Here's how the part is built. I have some questions about the finished solid (model axes, mm). Face numbers are marked on the shaded views. A direction names the side the tool comes from. Coordinates: 2 decimals unless noted, no trailing zeros. Write each loop counter-clockwise with the first axis right and the second up, starting at its lowest first coordinate (ties: lowest second). Pieces come first, ordered by that corner, then holes. Notation, with made-up numbers: (40, 23) - (85, 23) arc R21 cw to (85, 54) - close; hole circle Ø6 at (12.25, 11.25). An arc over 180 degrees is marked (long way). Answer in a Markdown table with one row per item. Add a question column.
Item 1: Imagine slicing it at C-C (y = 10.5). Please give me the cut outline in (x, z), plus the area to 3 significant figures.
Item 2: If I drill on probe 1 along X at (y, z) = (4, 4.55); probe 2 along Y at (x, z) = (3.5, 1.65); probe 3 along X at (y, z) = (-3.25, 0.2), over which ranges is the centre line in solid material (lowest first)? Write a range as from..to.
Item 3: Imagine slicing it at A-A (z = 1.5). Please give me the cut outline in (x, y).
Item 4: Which directions (+Z, -Z, +X, -X, +Y, -Y) give clear straight access to the entire face, cutting with the end or side of a thin tool? Please do the marked faces 1, 2 and 3.
Item 5: Imagine slicing it at B-B (x = -7.5). Please give me the cut outline in (y, z).
Item 6: I'm going to push flat-ended pins straight in: pin 1 (0.8 mm diameter, centred on y = 12.5, z = 0.5, fed in from +X); pin 2 (4 mm diameter, centred on x = -3.5, y = 1, fed in from -Z); pin 3 (1.3 mm diameter, centred on y = 10.5, z = 4, fed in from -X); pin 4 (2 mm diameter, centred on y = 9.5, z = 3.5, fed in from +X). Where does each tip first touch, or does it pass through?
from build123d import *

# Parameters (mm, degrees)
BOSS_EXTRUDE1_DEPTH = 5.5
BOSS_EXTRUDE2_DEPTH = 1


with BuildPart() as part:
    # Sketch1 → Boss-Extrude1 (new body)
    with BuildSketch(Plane.XY):
        Polygon((-14.173922558, 7.032133424), (-14.173922558, 1.032133424), (-7.173922558, 1.032133424), (-7.173922558, -5.967866576), (-1.173922558, -5.967866576), (-1.173922558, 1.032133424), (5.826077442, 1.032133424), (5.826077442, 7.032133424), (-1.173922558, 7.032133424), (-1.173922558, 14.032133424), (-7.173922558, 14.032133424), (-7.173922558, 7.032133424), align=None)
    extrude(amount=BOSS_EXTRUDE1_DEPTH)

    # Sketch2 → Boss-Extrude2 (add)
    with BuildSketch(Plane.XY):
        with BuildLine():
            Line((-15.873922558, 8.032133424), (-15.873922558, 0.032133424))
            ThreePointArc((-15.873922558, 0.032133424), (-15.668897304, -0.462841323), (-15.173922558, -0.667866576))
            Line((-15.173922558, -0.667866576), (-10.173922558, -0.667866576))
            ThreePointArc((-10.173922558, -0.667866576), (-9.254683742, -1.048627761), (-8.873922558, -1.967866576))
            Line((-8.873922558, -1.967866576), (-8.873922558, -6.967866576))
            ThreePointArc((-8.873922558, -6.967866576), (-8.668897304, -7.462841323), (-8.173922558, -7.667866576))
            Line((-8.173922558, -7.667866576), (-0.173922558, -7.667866576))
            ThreePointArc((-0.173922558, -7.667866576), (0.321052189, -7.462841323), (0.526077442, -6.967866576))
            Line((0.526077442, -6.967866576), (0.526077442, -1.967866576))
            ThreePointArc((0.526077442, -1.967866576), (0.906838627, -1.048627761), (1.826077442, -0.667866576))
            Line((1.826077442, -0.667866576), (6.826077442, -0.667866576))
            ThreePointArc((6.826077442, -0.667866576), (7.321052189, -0.462841323), (7.526077442, 0.032133424))
            Line((7.526077442, 0.032133424), (7.526077442, 8.032133424))
            ThreePointArc((7.526077442, 8.032133424), (7.321052189, 8.527108171), (6.826077442, 8.732133424))
            Line((6.826077442, 8.732133424), (1.826077442, 8.732133424))
            ThreePointArc((1.826077442, 8.732133424), (0.906838627, 9.112894608), (0.526077442, 10.032133424))
            Line((0.526077442, 10.032133424), (0.526077442, 15.032133424))
            ThreePointArc((0.526077442, 15.032133424), (0.321052189, 15.527108171), (-0.173922558, 15.732133424))
            Line((-0.173922558, 15.732133424), (-8.173922558, 15.732133424))
            ThreePointArc((-8.173922558, 15.732133424), (-8.668897304, 15.527108171), (-8.873922558, 15.032133424))
            Line((-8.873922558, 15.032133424), (-8.873922558, 10.032133424))
            ThreePointArc((-8.873922558, 10.032133424), (-9.254683742, 9.112894608), (-10.173922558, 8.732133424))
            Line((-10.173922558, 8.732133424), (-15.173922558, 8.732133424))
            ThreePointArc((-15.173922558, 8.732133424), (-15.668897304, 8.527108171), (-15.873922558, 8.032133424))
        make_face()
    extrude(amount=BOSS_EXTRUDE2_DEPTH)


solid = part.part
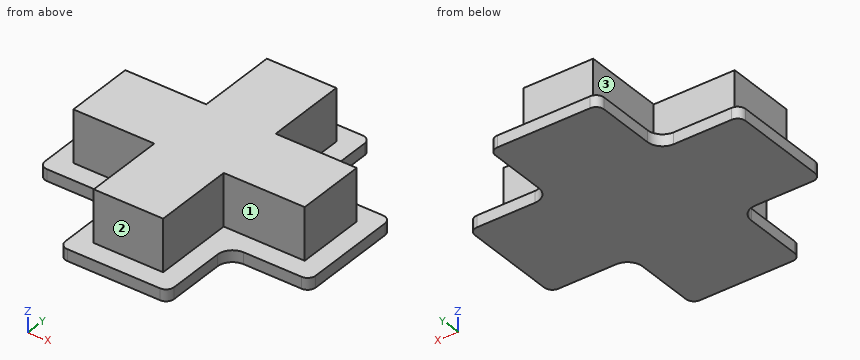
Here are the results:
| question | item | result |
|---|---|---|
| 1 | outline | (-8.87, 0) - (0.53, 0) - (0.53, 1) - (-1.17, 1) - (-1.17, 5.5) - (-7.17, 5.5) - (-7.17, 1) - (-8.87, 1) - close |
| 1 | area | 36.4 mm2 |
| 2 | probe 1 | x = -14.17..5.83 |
| 2 | probe 2 | y = 1.03..7.03 |
| 2 | probe 3 | x = -8.87..0.53 |
| 3 | outline | (-14.17, 1.03) - (-7.17, 1.03) - (-7.17, -5.97) - (-1.17, -5.97) - (-1.17, 1.03) - (5.83, 1.03) - (5.83, 7.03) - (-1.17, 7.03) - (-1.17, 14.03) - (-7.17, 14.03) - (-7.17, 7.03) - (-14.17, 7.03) - close |
| 4 | face 1 | +Z, +X, -Y |
| 4 | face 2 | +Z, +X, -X, -Y |
| 4 | face 3 | +Z, -X, +Y |
| 5 | outline | (-7.67, 0) - (15.73, 0) - (15.73, 1) - (7.03, 1) - (7.03, 5.5) - (1.03, 5.5) - (1.03, 1) - (-7.67, 1) - close |
| 6 | pin 1 | stops at x = 0.53 |
| 6 | pin 2 | stops at z = 0 |
| 6 | pin 3 | stops at x = -7.17 |
| 6 | pin 4 | stops at x = -1.17 |
